Read the model definition and answer for the solid it produces. Units are mm, in the model's axes. Round coordinates to 2 decimals unless told otherwise and drop trailing zeros. Write each loop counter-clockwise with the first axis right and the second up, starting at its lowest first coordinate (ties: lowest second). Pieces come first, ordered by that corner, then holes. Notation, with made-up numbers: (51, 54) - (103, 54) arc R12 ccw to (103, 65) - close; hole circle Ø4 at (70.25, -25.75). An arc over 180 degrees is marked (long way). Use one line per item in the form item = value. Start each with the question number.
1) Consider line 1 along Z through (x, y) = (0.5, 0.05); line 2 along Y through (x, z) = (-0.1, 11.75); line 3 along X through (y, z) = (0.1, 9.75). Determine where each line is inside the solid, lowest interval first. Write a range as from..to.
2) The part is cut by section A-A, the plane z = 4. Give the vertices of the cut face in (x, y), plus the area to 3 significant figures.
3) The part is cut by section B-B, the plane x = 0. Give the vertices of the cut face in (y, z).
4) The part is cut by section C-C, the plane z = -5. Give the vertices of the cut face in (x, y).
5) This flat-tipped pin is pushed along its axis until it touches: pin 1 (1.5 mm diameter, centred on x = 0, y = 0, fed in from +Z). Where does it stop, or does it pass through?
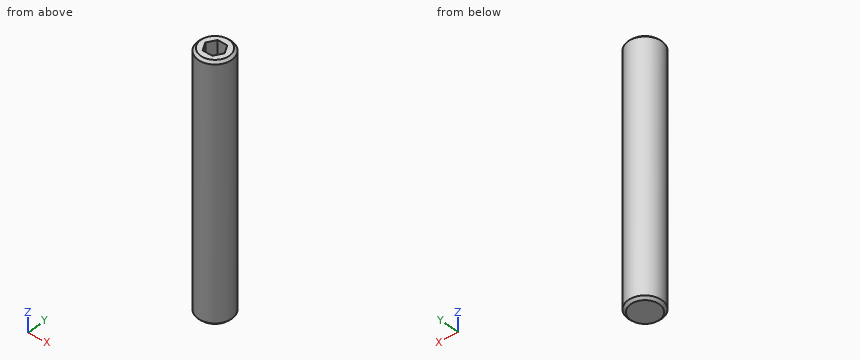
Solid Edge part; units mm, degrees
sketch "Sketch1" plane through (0, 0, 0) normal (0, 0, 1) x (1, 0, 0)
  circle A0 centre (0, 0) radius 2
extrude "Protrusion1" add sketch "Sketch1" along normal mid plane 30
chamfer "Chamfer1" distance 0.3 angle 45 2 edges at (-2, 0, -15) (-2, 0, 15)
sketch "Sketch2" plane through (0, 0, 15) normal (0, 0, 1) x (1, 0, 0)
  line L0 (-0.5774, 1) -> (0.5774, 1)
  line L1 (1.1547, 0) -> (0.5774, 1)
  line L2 (0.5774, -1) -> (1.1547, 0)
  line L3 (-0.5774, -1) -> (0.5774, -1)
  line L4 (-1.1547, 0) -> (-0.5774, -1)
  line L5 (-0.5774, 1) -> (-1.1547, 0)
extrude "Cutout1" cut sketch "Sketch2" against normal blind 15
properties part number "24100097"
Geometry results:
q1.line_1 = -15..0
q1.line_2 = -2..-1, 1..2
q1.line_3 = -2..-1.1, 1.1..2
q2.outline = circle Ø4 at (0, 0); hole (-1.15, 0) - (-0.58, -1) - (0.58, -1) - (1.15, 0) - (0.58, 1) - (-0.58, 1) - close
q2.area = 9.10 mm2
q3.outline = (-2, -14.7) - (-1.7, -15) - (1.7, -15) - (2, -14.7) - (2, 14.7) - (1.7, 15) - (1, 15) - (1, 0) - (-1, 0) - (-1, 15) - (-1.7, 15) - (-2, 14.7) - close
q4.outline = circle Ø4 at (0, 0)
q5.pin_1 = 0
